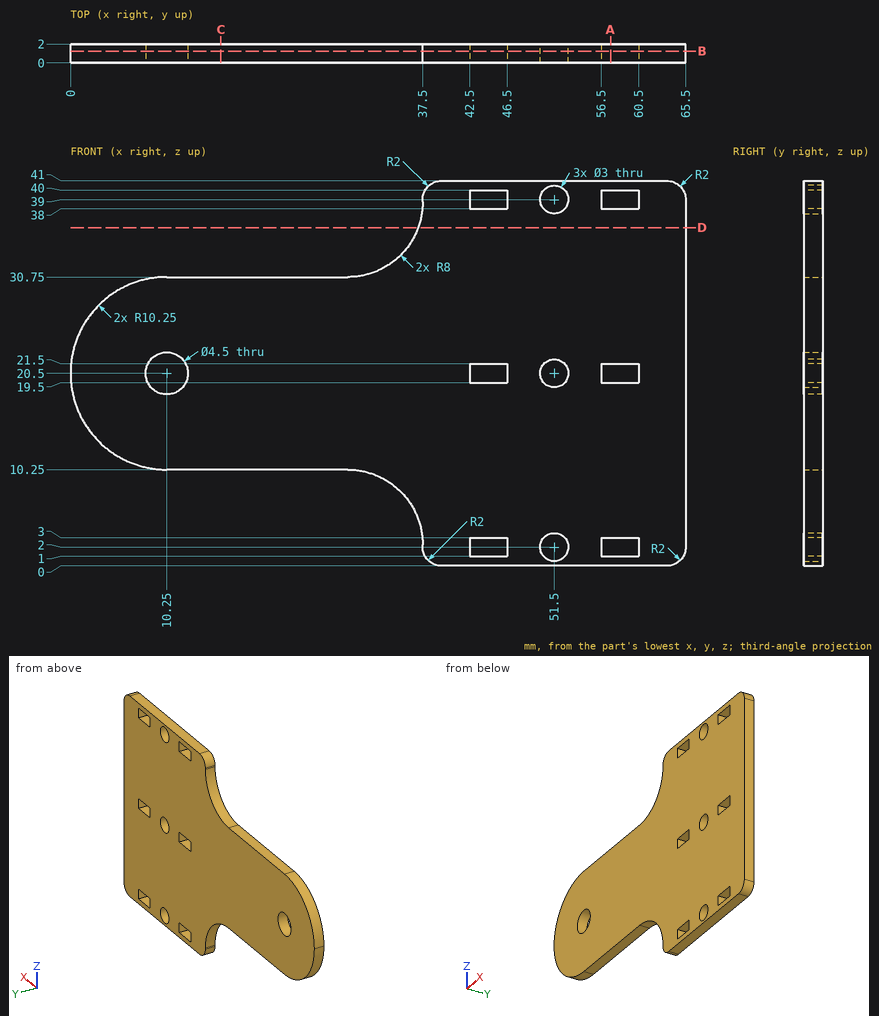
Geometry: see drawing. Coordinates: mm, zero at the bounding-box minimum. Coordinates: 2 decimals unless noted, no trailing zeros. Loops run counter-clockwise (first coordinate to the right, second up) from the corner with the lowest first, then second, coordinate; pieces in that order, holes last. Notation, with made-up numbers: M 67,41.25 L 108,41.25 A17 cw 108,51.25 Z; hole C -5,66 d11. An arc over 180 degrees is marked long. Answer in a Markdown table with one row per item.
1. Section D-D, the plane z = 36. Output: boundary loops of the cut face in (x, y).
Response:
| item | result |
|---|---|
| outline | M 37.01,0 L 65.5,0 L 65.5,2 L 37.01,2 Z |
2. Section A-A, the plane x = 57.5. Output: boundary loops of the cut face in (y, z), then the cut area to 3 significant figures.
Response:
| item | result |
|---|---|
| outline | M 0,0 L 2,0 L 2,1 L 0,1 Z; M 0,3 L 2,3 L 2,19.5 L 0,19.5 Z; M 0,21.5 L 2,21.5 L 2,38 L 0,38 Z; M 0,40 L 2,40 L 2,41 L 0,41 Z |
| area | 70.0 mm2 |
3. Section C-C, the plane x = 16. Output: boundary loops of the cut face in (y, z), then the cut area to 3 significant figures.
Response:
| item | result |
|---|---|
| outline | M 0,10.25 L 2,10.25 L 2,30.75 L 0,30.75 Z |
| area | 41.0 mm2 |
4. Section B-B, the plane y = 1.25. Count the separate pieces of the cut face and the enclosed holes in it, then the cut area to 3 significant figures.
Response:
| item | result |
|---|---|
| separate pieces | 1 |
| enclosed holes | 10 |
| area | 1,810 mm2 |
5. First-contact query: pin 1 (0.6 mm diameter, centred on y = 1, z = 1.5, fed in from +X); pin 2 (0.6 mm diameter, centred on x = 19, y = 1.5, fed in from -Z); pin 3 (0.6 mm diameter, centred on y = 1, z = 2, fed in from -X). Flat tips, straight axial feed; report the tip coordinate or a pass-through.
Response:
| item | result |
|---|---|
| pin 1 | stops at x = 65.49 |
| pin 2 | stops at z = 10.25 |
| pin 3 | stops at x = 37.5 |
6. Material intervals for line 1 (X direction, y = 1.55, z = 20.5); line 2 (X direction, y = 0.75, z = 2); line 3 (Z direction, x = 10, y = 0.6), sorted ascending.
Response:
| item | result |
|---|---|
| line 1 | x = 0 to 8, 12.5 to 42.5, 46.5 to 50, 53 to 56.5, 60.5 to 65.5 |
| line 2 | x = 37.5 to 42.5, 46.5 to 50, 53 to 56.5, 60.5 to 65.5 |
| line 3 | z = 10.25 to 18.26, 22.74 to 30.75 |
